Source: CAD feature listing. Evaluate the final solid. Frame: model axes, mm. A direction names the side the tool comes from. Coordinates: 2 decimals unless noted, no trailing zeros. Order: outer loops, then holes, each group sorted by start corner. A loop starts at its lowest first (then second) coordinate and runs counter-clockwise, first axis right, second up.
Autodesk Inventor part; units mm, degrees
ref_plane "YZ Plane" through (0, 0, 0) normal (1, 0, 0) x (0, 1, 0)
ref_plane "XZ Plane" through (0, 0, 0) normal (0, 1, 0) x (-1, 0, 0)
ref_plane "XY Plane" through (0, 0, 0) normal (0, 0, 1) x (1, 0, 0)
sketch "Эскиз1" plane through (0, 0, 0) normal (0, 1, 0) x (-1, 0, 0)
  line L0 (40, 17.5) -> (-40, 17.5)
  line L1 (-50, 7.5) -> (-50, -7.5)
  line L2 (-40, -17.5) -> (40, -17.5)
  line L3 (50, -7.5) -> (50, 7.5)
  line L4 (0, 0) -> (103.6754, 0) construction
  line L5 (0, 0) -> (0, -121.5896) construction
  line L6 (14.4533, -17.5) -> (50.9438, -61.6825)
  circle A0 centre (57.3118, -69.3928) radius 10
  arc A1 (53.3569, -60.2081) -> (22.4906, -17.5) centre (-76.5583, -121.5932) ccw
  line L7 (0, 0) -> (119.3987, -22.9778) construction
  arc A2 (8.22, -17.5) -> (49.04, -63.7734) centre (133.8701, 52.2004) ccw
  arc A3 (40, -17.5) -> (50, -7.5) centre (40, -7.5) ccw
  arc A4 (50, 7.5) -> (40, 17.5) centre (40, 7.5) ccw
  arc A5 (-40, 17.5) -> (-50, 7.5) centre (-40, 7.5) ccw
  arc A6 (-50, -7.5) -> (-40, -17.5) centre (-40, -7.5) ccw
  line L8 (-14.4533, -17.5) -> (-50.9438, -61.6825)
  circle A7 centre (-57.3118, -69.3928) radius 10
  arc A8 (-22.4906, -17.5) -> (-53.3569, -60.2081) centre (76.5583, -121.5932) ccw
  arc A9 (-49.04, -63.7734) -> (-8.22, -17.5) centre (-133.8701, 52.2004) ccw
  line L9 (0, 0) -> (0, 121.5896) construction
  line L10 (14.4533, 17.5) -> (50.9438, 61.6825)
  circle A10 centre (57.3118, 69.3928) radius 10
  arc A11 (22.4906, 17.5) -> (53.3569, 60.2081) centre (-76.5583, 121.5932) ccw
  arc A12 (49.04, 63.7734) -> (8.22, 17.5) centre (133.8701, -52.2004) ccw
  circle A13 centre (-57.3118, 69.3928) radius 10
  arc A14 (-53.3569, 60.2081) -> (-22.4906, 17.5) centre (76.5583, 121.5932) ccw
  line L11 (-14.4533, 17.5) -> (-50.9438, 61.6825)
  arc A15 (-8.22, 17.5) -> (-49.04, 63.7734) centre (-133.8701, -52.2004) ccw
  point P0 (50, 17.5)
  point P1 (-50, -17.5)
  point P2 (50, -17.5)
  point P3 (-22.4906, -17.5)
  point P4 (-8.22, -17.5)
  point P5 (22.4906, 17.5)
  point P6 (8.22, 17.5)
  point P7 (-8.22, 17.5)
  point P8 (-22.4906, 17.5)
  dimension "d0" = 35
  dimension "d1" = 100
  dimension "d2" = 50
  dimension "d3" = 35
  dimension "d4" = 17.5
  dimension "d5" = 80
  dimension "d6" = 20
  dimension "d7" = 10
  dimension "d8" = 10
extrude "Выдавливание1" add sketch "Эскиз1" along normal blind 4
sketch "Эскиз2" plane through (0, 4, 0) normal (0, 1, 0) x (1, 0, 0)
  line L0 (-25, -12.5) -> (-15, -12.5)
  line L1 (-15, -12.5) -> (-15, -8.5)
  line L2 (-15, -8.5) -> (-25, -8.5)
  line L3 (-25, -8.5) -> (-25, -12.5)
  line L4 (-50, 7.5) -> (-50, -7.5)
  line L5 (-40, -17.5) -> (-22.4906, -17.5)
  line L6 (0, 0) -> (-53.5692, 0) construction
  line L7 (0, 0) -> (0, -51.6418) construction
  line L8 (-25, 12.5) -> (-15, 12.5)
  line L9 (-15, 12.5) -> (-15, 8.5)
  line L10 (-15, 8.5) -> (-25, 8.5)
  line L11 (-25, 8.5) -> (-25, 12.5)
  line L12 (-40, 17.5) -> (-22.4906, 17.5)
  line L13 (0, 0) -> (0, 51.6418) construction
  line L14 (25, -12.5) -> (15, -12.5)
  line L15 (15, -12.5) -> (15, -8.5)
  line L16 (15, -8.5) -> (25, -8.5)
  line L17 (25, -8.5) -> (25, -12.5)
  line L18 (25, 12.5) -> (15, 12.5)
  line L19 (15, 12.5) -> (15, 8.5)
  line L20 (15, 8.5) -> (25, 8.5)
  line L21 (25, 8.5) -> (25, 12.5)
  dimension "d11" = 4
  dimension "d12" = 10
  dimension "d13" = 25
  dimension "d14" = 5
extrude "Выдавливание2" cut sketch "Эскиз2" against normal blind 4
sketch "Эскиз3" plane through (0, 4, 0) normal (0, 1, 0) x (1, 0, 0)
  line L0 (-40, -4.453) -> (-44, -4.453)
  line L1 (-44, -4.453) -> (-44, 5.547)
  line L2 (-44, 5.547) -> (-40, 5.547)
  line L3 (-40, 5.547) -> (-40, -4.453)
  line L4 (-50, 7.5) -> (-50, -7.5)
  line L5 (0, 0) -> (0, 42.0711) construction
  line L6 (40, -4.453) -> (44, -4.453)
  line L7 (44, -4.453) -> (44, 5.547)
  line L8 (44, 5.547) -> (40, 5.547)
  line L9 (40, 5.547) -> (40, -4.453)
  dimension "d17" = 10
  dimension "d18" = 4
  dimension "d19" = 10
extrude "Выдавливание3" cut sketch "Эскиз3" against normal blind 4
properties part number "Dron"
1. Section query C-C, the plane x = 17. Output: boundary loops of the cut face in (y, z).
2. Section query B-B, the plane x = 56.5. Output: boundary loops of the cut face in (y, z).
3. Material intervals for line 1 along X through (y, z) = (1.6, -5.5); line 2 along Z through (x, y) = (-17.5, 1.45); line 3 along Z through (x, y) = (-24, 1.9), sorted ascending.
4. Access query for faces 1 (the flat face through (25, 2, 10)), 2 (the flat face through (-31, 2, -17.5)), 3 (the cylindrical face through (47.15, 1.97, 14.49)), 4 (the flat face through (0, 2, 17.5)). Directions: +Z, -Z, +X, -X, +Y, -Y. A direction counts if a zero-diameter tool reaches every point of the face in a straight line with its end or side. Return the directions, or none.
5. Section query A-A, the plane z = -48. Output: boundary loops of the cut face in (x, y).
6. Contact query for flat-ended pins moving along their axis: P1, Ø1.5, axis at x = -49.5, y = 3, coming from the +Z side; P2, Ø12, axis at x = 18, z = -24, coming from the -Y side; P3, Ø1, axis at y = 1, z = 12.5, coming from the +X side; P4, Ø1.2, axis at x = 20, y = 1, coming from the +Z side. Output: stop coordinate, or through.
7. Section query D-D, the plane x = -5.5. Output: boundary loops of the cut face in (y, z), plus the area to 3 significant figures.
Answer key:
1. outline: (0, -31.39) - (4, -31.39) - (4, -12.5) - (0, -12.5) - close; (0, -8.5) - (4, -8.5) - (4, 8.5) - (0, 8.5) - close; (0, 12.5) - (4, 12.5) - (4, 31.39) - (0, 31.39) - close
2. outline: (0, -79.36) - (4, -79.36) - (4, -59.43) - (0, -59.43) - close; (0, 59.43) - (4, 59.43) - (4, 79.36) - (0, 79.36) - close
3. line 1: x = -50 to -44, -40 to 40, 44 to 50
3. line 2: z = -32.09 to -12.5, -8.5 to 8.5, 12.5 to 32.09
3. line 3: z = -40.4 to -18.96, -17.5 to -12.5, -8.5 to 8.5, 12.5 to 17.5, 18.96 to 40.4
4. face 1: +Y, -Y
4. face 2: -X, +Y, -Y
4. face 3: +X, +Y, -Y
4. face 4: +Z, +Y, -Y
5. outline: (-46.85, 0) - (-30.88, 0) - (-30.88, 4) - (-46.85, 4) - close; (30.88, 0) - (46.85, 0) - (46.85, 4) - (30.88, 4) - close
6. P1: stops at z = 76.47
6. P2: stops at y = 0
6. P3: stops at x = 48.93
6. P4: stops at z = 36.21
7. outline: (0, -17.5) - (4, -17.5) - (4, 17.5) - (0, 17.5) - close
7. area: 140 mm2
